from build123d import *

# Parameters (mm, degrees)
SKETCH1_R           = 4.6
BOSS_EXTRUDE1_DEPTH = 7.3
SKETCH2_R           = 2.1
BOSS_EXTRUDE2_DEPTH = 7.8
BOSS_EXTRUDE3_START = -7.3
SKETCH3_W           = 0.76
SKETCH3_H           = 0.7
BOSS_EXTRUDE3_DEPTH = 2.2


with BuildPart() as part:
    # Sketch1 → Boss-Extrude1 (new body)
    with BuildSketch(Plane.XY):
        Circle(SKETCH1_R)
    extrude(amount=BOSS_EXTRUDE1_DEPTH)

    # Sketch2 → Boss-Extrude2 (add)
    with BuildSketch(Plane.XY.offset(7.3)):
        Circle(SKETCH2_R)
    extrude(amount=BOSS_EXTRUDE2_DEPTH)

    # Sketch3 → Boss-Extrude3 (add)
    with BuildSketch(Plane.XY.offset(7.3).offset(BOSS_EXTRUDE3_START)):
        with Locations((0.008541009, 4.88)):
            Rectangle(SKETCH3_W, SKETCH3_H)
    extrude(amount=BOSS_EXTRUDE3_DEPTH)


solid = part.part
Check sheet for the modelled part. Datum: model origin and axes. Units: mm. A direction names the side the tool comes from. Round coordinates to 2 decimals unless told otherwise and drop trailing zeros. Loops run counter-clockwise (first coordinate to the right, second up) from the corner with the lowest first, then second, coordinate; pieces in that order, holes last. Notation, with made-up numbers: (-2, -7.5) - (29, -7.5) arc R15 ccw to (29, 7.5) - close; hole circle Ø6 at (-25, 89.5). An arc over 180 degrees is marked (long way). Answer as CSV lines item,"result". Start each with the question number.
Item 1: Scan lines: line 1 (Z direction, x = -2, y = -2.5); line 2 (Y direction, x = -3.5, z = 4); line 3 (Y direction, x = -0.75, z = 11). Record each from-to range of solid material in increasing order. Write a range as [from, to].
Item 2: Section check D-D (y = -1.5). Record the boundary of the cut face in (x, z), and give its area (3 significant figures).
Item 3: Set-up check for faces 1 (the flat face through (-1.1, -2, 7.3)), 2 (the flat face through (0, 0, 0)): record each of +Z, -Z, +X, -X, +Y, -Y from which the full face is reachable in a straight line by a thin tool's end or side.
Item 4: Section check B-B (y = 0.75). Record the boundary of the cut face in (x, z), and give its area (3 significant figures).
Item 5: Section check A-A (x = 0). Record the boundary of the cut face in (y, z).
Item 6: Release check for a two-part mould opening along X. For faces 3 (the cylindrical face through (-3.65, -2.8, 3.6)), 4 (the flat face through (0, 0, 15.1)) record: +X half, -X half, draft (parallel to the pull), parting line (faces both ways), or undercut.
Item 7: Section check C-C (z = 1.75). Record the boundary of the cut face in (x, y), and give its area (3 significant figures).
Item 8: Depth check by flat-ended pin: P1, Ø0.7, axis at y = 4.5, z = 1, coming from the +X side; P2, Ø0.5, axis at y = 5, z = 1, coming from the -X side; P3, Ø3, axis at y = -1, z = 10.5, coming from the +X side; P4, Ø2, axis at x = 0, y = 3, coming from the -Z side. Enter the tip coordinate at first touch or a pass-through.
Report:
1,line 1,"z = [0, 7.3]"
1,line 2,"y = [-2.98, 2.98]"
1,line 3,"y = [-1.96, 1.96]"
2,outline,"(-4.35, 0) - (4.35, 0) - (4.35, 7.3) - (1.47, 7.3) - (1.47, 15.1) - (-1.47, 15.1) - (-1.47, 7.3) - (-4.35, 7.3) - close"
2,area,"86.4 mm2"
3,face 1,"+Z"
3,face 2,"-Z, +X, -X, +Y, -Y"
4,outline,"(-4.54, 0) - (4.54, 0) - (4.54, 7.3) - (1.96, 7.3) - (1.96, 15.1) - (-1.96, 15.1) - (-1.96, 7.3) - (-4.54, 7.3) - close"
4,area,"96.9 mm2"
5,outline,"(-4.6, 0) - (5.23, 0) - (5.23, 2.2) - (4.6, 2.2) - (4.6, 7.3) - (2.1, 7.3) - (2.1, 15.1) - (-2.1, 15.1) - (-2.1, 7.3) - (-4.6, 7.3) - close"
6,face 3,"parting line"
6,face 4,"draft"
7,outline,"(-0.37, 4.58) arc R4.6 ccw (long way) to (0.39, 4.58) - (0.39, 5.23) - (-0.37, 5.23) - close"
7,area,"67.0 mm2"
8,P1,"stops at x = 1.98"
8,P2,"stops at x = -0.37"
8,P3,"stops at x = 2.1"
8,P4,"stops at z = 0"
